```python
from build123d import *

# Parameters (mm, degrees)
EXTRUDE1_DEPTH             = 1.6
SKETCH2_W                  = 9.5
SKETCH2_H                  = 1.6
SKETCH2_W_2                = 41
EXTRUDE2_DEPTH             = 25
FILLET2_R                  = 0.4
FILLET3_R                  = 2
F_3_7_3_7_DIAMETER_HOLE1_D = 3.7
SKETCH4_R                  = 1.6
CUT_EXTRUDE2_DEPTH         = 2.6
SKETCH5_R                  = 4
CUT_EXTRUDE3_DEPTH         = 2.6
SKETCH5_3_R                = 1.85
CUT_EXTRUDE4_DEPTH         = 2.6
CIRPATTERN1_COUNT          = 4
SKETCH5_4_R                = 1.85
CUT_EXTRUDE5_DEPTH         = 10
CIRPATTERN2_COUNT          = 4


with BuildPart() as part:
    # Sketch1 → Extrude1 (new body)
    with BuildSketch(Plane(origin=(0, 0, 0), x_dir=(1, 0, 0), z_dir=(0, 1, 0))):
        Polygon((-30, -10.6), (-30, 10.6), (-20.5, 10.6), (-20.5, 18.83069384), (20.5, 18.83069384), (20.5, 10.6), (30, 10.6), (30, -10.6), (20.5, -10.6), (20.5, -6.588025881), (17.5, -6.588025881), (17.5, -13.838875216), (-17.5, -13.838875216), (-17.5, -6.588025881), (-20.5, -6.588025881), (-20.5, -10.6), align=None)
    extrude(amount=EXTRUDE1_DEPTH)

    # Sketch2 → Extrude2 (add)
    with BuildSketch(Plane(origin=(0, 1.6, 0), x_dir=(1, 0, 0), z_dir=(0, 1, 0))):
        with Locations((-25.25, -9.8)):
            Rectangle(SKETCH2_W, SKETCH2_H)
        with Locations((25.25, -9.8)):
            Rectangle(SKETCH2_W, SKETCH2_H)
        with Locations((0, 18.03069384)):
            Rectangle(SKETCH2_W_2, SKETCH2_H)
    extrude(amount=EXTRUDE2_DEPTH)

    # Fillet2
    fillet2_edges = [part.edges().sort_by_distance(p)[0] for p in [
        (-25.25, 1.6, 9),
        (25.25, 1.6, 9),
        (0, 1.6, -17.23069384),
    ]]
    fillet(fillet2_edges, radius=FILLET2_R)

    # Fillet3
    fillet3_edges = [part.edges().sort_by_distance(p)[0] for p in [
        (-30, 0.8, -10.6),
        (-17.5, 0.8, 13.838875216),
        (30, 0.8, -10.6),
        (20.5, 26.6, 9.8),
        (30, 26.6, 9.8),
        (20.5, 26.6, -18.03069384),
        (-20.5, 26.6, -18.03069384),
        (-30, 26.6, 9.8),
        (-20.5, 26.6, 9.8),
        (-25.25, 0, 10.6),
        (25.25, 0, 10.6),
        (0, 0, -18.83069384),
        (17.5, 0.8, 13.838875216),
    ]]
    fillet(fillet3_edges, radius=FILLET3_R)

    # 3.7 _3.7_ Diameter Hole1 (through all)
    with Locations(Plane.XY.offset(10.6)):
        with Locations((-23.75, 21.6), (-23.75, 11.6), (23.75, 11.6), (23.75, 21.6)):
            Hole(F_3_7_3_7_DIAMETER_HOLE1_D / 2)

    # Sketch4 → Cut-Extrude2 (cut, through all)
    with BuildSketch(Plane.XY.offset(-17.23069384)):
        with Locations((10, 17.09445923)):
            Circle(SKETCH4_R)
        with Locations((-10, 17.09445923)):
            Circle(SKETCH4_R)
    extrude(amount=-CUT_EXTRUDE2_DEPTH, mode=Mode.SUBTRACT)

    # Sketch5 → Cut-Extrude3 (cut, through all)
    with BuildSketch(Plane(origin=(0, 1.6, 0), x_dir=(1, 0, 0), z_dir=(0, 1, 0))):
        with Locations((8, 0)):
            Circle(SKETCH5_R)
        with Locations((-8, 0)):
            Circle(SKETCH5_R)
    extrude(amount=-CUT_EXTRUDE3_DEPTH, mode=Mode.SUBTRACT)

    # Sketch5_3 → Cut-Extrude4 (cut, through all)
    with BuildSketch(Plane(origin=(0, 1.6, 0), x_dir=(1, 0, 0), z_dir=(0, 1, 0))):
        with Locations((8, 8)):
            Circle(SKETCH5_3_R)
    cut_extrude4 = extrude(amount=-CUT_EXTRUDE4_DEPTH, mode=Mode.SUBTRACT)

    # CirPattern1: Cut-Extrude4 ×4 about axis
    cirpattern1_axis = Axis((8, 0, 0), (0, 1, 0))
    for i in range(1, CIRPATTERN1_COUNT):
        add(cut_extrude4.rotate(cirpattern1_axis, i * 360 / CIRPATTERN1_COUNT), mode=Mode.SUBTRACT)

    # Sketch5_4 → Cut-Extrude5 (cut)
    with BuildSketch(Plane(origin=(0, 1.6, 0), x_dir=(1, 0, 0), z_dir=(0, 1, 0))):
        with Locations((-8, 8)):
            Circle(SKETCH5_4_R)
    cut_extrude5 = extrude(amount=-CUT_EXTRUDE5_DEPTH, mode=Mode.SUBTRACT)

    # CirPattern2: Cut-Extrude5 ×4 about axis
    cirpattern2_axis = Axis((-8, 0, 0), (0, 1, 0))
    for i in range(1, CIRPATTERN2_COUNT):
        add(cut_extrude5.rotate(cirpattern2_axis, i * 360 / CIRPATTERN2_COUNT), mode=Mode.SUBTRACT)


solid = part.part
```
Geometry: final body of the model. Coordinates: model frame, mm. A direction names the side the tool comes from. Coordinates: 2 decimals unless noted, no trailing zeros. Loops run counter-clockwise (first coordinate to the right, second up) from the corner with the lowest first, then second, coordinate; pieces in that order, holes last. Notation, with made-up numbers: M 20.5,3 L 48.5,3 A17 cw 48.5,13 Z; hole C -6,-38.75 d2. An arc over 180 degrees is marked long. Put each result on its own line as item: value.
(1) Access query for faces 4 (the face through (17.5, 1, 9)), 5 (the face through (24, 1, -10.6)), 6 (the face through (-20.5, 9.5, -17.4)). Directions: +Z, -Z, +X, -X, +Y, -Y. A direction counts if a zero-diameter tool reaches every point of the face in a straight line with its end or side. Return the directions, or none.
Answer sheet:
face 4: +Z, +Y, -Y
face 5: -Z, +X, +Y, -Y
face 6: -Z, -X, +Y, -Y
(2) Cut plane A-A on x = 0. Return the cut outline in (y, z), then the cut area to 3 significant figures.
Answer sheet:
outline: M 0,-16.83 A2 ccw 2,-18.83 L 26.6,-18.83 L 26.6,-17.23 L 2,-17.23 A0.4 cw 1.6,-16.83 L 1.6,-1.85 L 0,-1.85 Z; M 0,1.85 L 1.6,1.85 L 1.6,13.84 L 0,13.84 Z
area: 85.5 mm^2
(3) Cut plane C-C on x = -23.75. Return the cut outline in (y, z), then the cut area to 3 significant figures.
Answer sheet:
outline: M 0,-10.6 L 1.6,-10.6 L 1.6,8.6 A0.4 cw 2,9 L 9.75,9 L 9.75,10.6 L 2,10.6 A2 ccw 0,8.6 Z; M 13.45,9 L 19.75,9 L 19.75,10.6 L 13.45,10.6 Z; M 23.45,9 L 26.6,9 L 26.6,10.6 L 23.45,10.6 Z
area: 61.3 mm^2
(4) Cut plane B-B on y = 9. Return the cut outline in (x, z), then the cut area to 3 significant figures.
Answer sheet:
outline: M -30,9 L -20.5,9 L -20.5,10.6 L -30,10.6 Z; M -20.5,-18.83 L 20.5,-18.83 L 20.5,-17.23 L -20.5,-17.23 Z; M 20.5,9 L 30,9 L 30,10.6 L 20.5,10.6 Z
area: 96.0 mm^2
(5) Draft query along X for faces 1 (the face through (25, 26.6, 10)), 2 (the face through (17.834, 0.811, -0.241)), 3 (the face through (30, 6.8, 9.5)). Return one class per face: pulls with the +X half, pulls with the -X half, needs draft (parallel to the pull), parting line crosses it, or undercut.
Answer sheet:
face 1: needs draft
face 2: undercut
face 3: pulls with the +X half
(6) First-contact query: pin 1 (4 mm diameter, centred on x = -1.5, z = 7, fed in from +Y); pin 2 (4 mm diameter, centred on x = -10, y = 10, fed in from +Z); pin 3 (6.5 mm diameter, centred on y = 7.5, z = -16.5, fed in from -X). Flat tips, straight axial feed; report the tip coordinate or a pass-through.
Answer sheet:
pin 1: stops at y = 1.6
pin 2: stops at z = -17.23
pin 3: stops at x = -20.5
(7) Cut plane D-D on z = -8. Return the cut outline in (x, y).
Answer sheet:
outline: M -30,0 L -9.85,0 L -9.85,1.6 L -30,1.6 Z; M -6.15,0 L 6.15,0 L 6.15,1.6 L -6.15,1.6 Z; M 9.85,0 L 30,0 L 30,1.6 L 9.85,1.6 Z
(8) Material intervals for probe 1 along X at (y, z) = (0.8, 0); probe 2 along X at (y, z) = (1.25, 12); probe 3 along Z at (x, y) = (26.5, 20.5), sorted ascending.
Answer sheet:
probe 1: x = -30 to -17.85, -14.15 to -12, -4 to -1.85, 1.85 to 4, 12 to 14.15, 17.85 to 30
probe 2: x = -17.49 to 17.49
probe 3: z = 9 to 10.6
